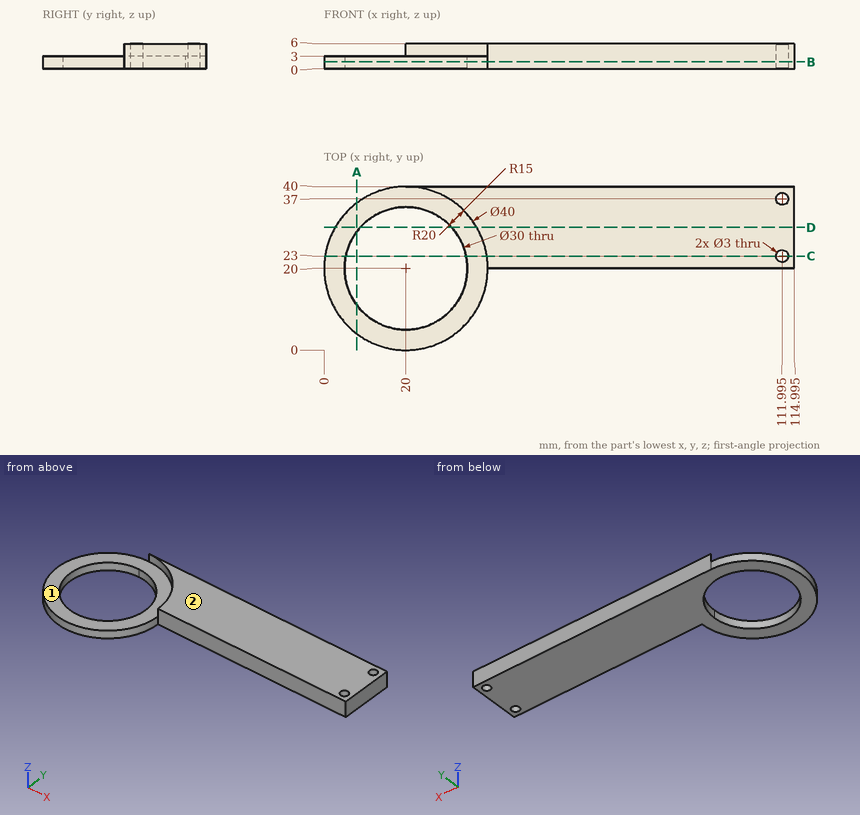
Can you work these out from the drawing? Everything is in mm from the part's minimum corner. A direction names the side the tool comes from. Coordinates: 2 decimals unless noted, no trailing zeros. Loops run counter-clockwise (first coordinate to the right, second up) from the corner with the lowest first, then second, coordinate; pieces in that order, holes last. Notation, with made-up numbers: M 13.5,51 L 67.5,51 A31 ccw 67.5,77 Z; hole C -0.5,-11.5 d3. An arc over 180 degrees is marked long. Put each result on its own line as item: value. Start each with the question number.
(1) Suppose I cut it at A-A on x = 8. Please give me the cut outline in (y, z).
(2) Will these pins go through, and if not, where does the flat tip stop? P1, Ø12, axis at x = 46, y = 11.5, coming from the +Z side; P2, Ø20, axis at x = 11, y = 25, coming from the +Z side; P3, Ø3, axis at x = 82, z = 2.5, coming from the -Y side.
(3) Suppose I cut it at B-B on z = 1.6. Please give me the cut outline in (x, y) (1 decimal).
(4) Suppose I cut it at D-D on y = 30. Please give me the cut outline in (x, z) (1 decimal), then the cut area to 3 significant figures.
(5) For the marked faces 1 and 2, which set-ups out of +Z, -Z, +X, -X, +Y, -Y let a thin tool reach every point of the face, with its end or its side?
(6) Suppose I cut it at C-C on y = 23. Please give me the cut outline in (x, z) (1 decimal), then the cut area to 3 significant figures.
(7) I need wall thicknesses on line 1 (Y direction, x = 97.5, z = 4.85); line 2 (Y direction, x = 19, z = 1.4) (1 decimal); line 3 (X direction, y = 29, z = 0.3) (1 decimal). Which ranges of each line are inside material? Lowest first, please. Write a range as from..to.
Solutions:
1. outline: M 4,0 L 11,0 L 11,3 L 4,3 Z; M 29,0 L 36,0 L 36,3 L 29,3 Z
2. P1: passes through
2. P2: stops at z = 3
2. P3: stops at y = 20
3. outline: M 20,40 A20 ccw long 40,20 L 115,20 L 115,40 Z; hole C 20,20 d30; hole C 112,23 d3; hole C 112,37 d3
4. outline: M 2.7,0 L 8.8,0 L 8.8,3 L 2.7,3 Z; M 31.2,0 L 115,0 L 115,6 L 37.3,6 L 37.3,3 L 31.2,3 Z
4. area: 503 mm2
5. face 1: +Z, -X, -Y
5. face 2: +Z, +X, -X, +Y, -Y
6. outline: M 0.2,0 L 5.3,0 L 5.3,3 L 0.2,3 Z; M 34.7,0 L 110.5,0 L 110.5,6 L 39.8,6 L 39.8,3 L 34.7,3 Z; M 113.5,0 L 115,0 L 115,6 L 113.5,6 Z
6. area: 464 mm2
7. line 1: y = 20..40
7. line 2: y = 0..5, 35..40
7. line 3: x = 2.1..8, 32..115
